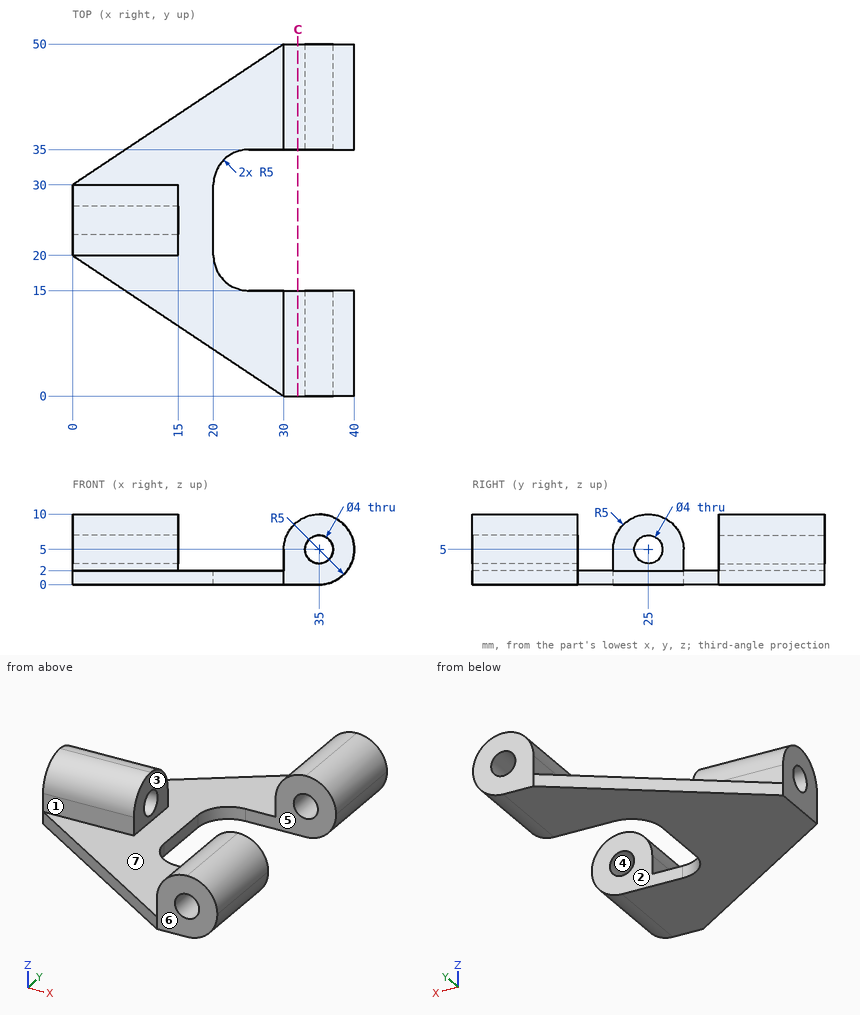
Verification items for this drawing (mm, ordinates from the low corner). A direction names the side the tool comes from. Round coordinates to 2 decimals unless told otherwise and drop trailing zeros. Order: outer loops, then holes, each group sorted by start corner. A loop starts at its lowest first (then second) coordinate and runs counter-clockwise, first axis right, second up. Notation, with made-up numbers: M 56.5,-33 L 91.5,-33 A24 cw 91.5,-15 Z; hole C 53,6.5 d3. An arc over 180 degrees is marked long. Answer in a Markdown table with one row per item. Add a question column.
Item 1: Draft check along Y on the marked faces 5, 6 and 7. Enter one of: released by +Y, released by -Y, zero draft, split by the parting line, or undercut.
Item 2: Depth check by flat-ended pin: pin 1 Ø1.5 at (x, z) = (8, 3.5) entering from +Y; pin 2 Ø15 at (x, y) = (13.5, 15.5) entering from +Z; pin 3 Ø2.5 at (x, z) = (35, 5) entering from -Y; pin 4 Ø2 at (y, z) = (27, 1.5) entering from +X. Enter the tip coordinate at first touch or a pass-through.
Item 3: Sectioned sample at C-C, the plane x = 32. Enter the section's corners in (y, z).
Item 4: Set-up check for the marked faces 1, 2, 3 and 4: record each of +Z, -Z, +X, -X, +Y, -Y from which the full face is reachable in a straight line by a thin tool's end or side.
Item 5: Material ranges on L1, parallel to Y at x = 35.5, z = 7; L2, parallel to Z at x = 5, y = 25; L3, parallel to Z at x = 28, y = 46, recorded low to high. Write a range as [from, to].
Filled in:
| question | item | result |
|---|---|---|
| 1 | face 5 | undercut |
| 1 | face 6 | released by -Y |
| 1 | face 7 | zero draft |
| 2 | pin 1 | stops at y = 30 |
| 2 | pin 2 | stops at z = 9.58 |
| 2 | pin 3 | passes through |
| 2 | pin 4 | stops at x = 20 |
| 3 | outline | M 0,0 L 15,0 L 15,9 L 0,9 Z; M 35,0 L 50,0 L 50,9 L 35,9 Z |
| 4 | face 1 | +Z, +X, -X, -Y |
| 4 | face 2 | +Z, -Z, +X |
| 4 | face 3 | +Z, +X, +Y, -Y |
| 4 | face 4 | +Y, -Y |
| 5 | L1 | y = [0, 15], [35, 50] |
| 5 | L2 | z = [0, 3], [7, 10] |
| 5 | L3 | z = [0, 2] |
